Can you work these out from the model? Positions are in its coordinate system, mm. Face numbers are marked on the shaded views. A direction names the side the tool comes from. Round coordinates to 2 decimals unless told otherwise and drop trailing zeros. Order: outer loops, then holes, each group sorted by start corner. A loop starts at its lowest first (then second) coordinate and runs counter-clockwise, first axis right, second up. Notation, with made-up numbers: (4, 74) -> (53, 74) arc R31 ccw to (53, 102) -> close; hole circle Ø10 at (83, 36). An arc over 180 degrees is marked (long way). Use a Markdown table: item, result. Add a question column.
Q1. I need wall thicknesses on line 1 along X through (y, z) = (-21, 76.5); line 2 along Y through (x, z) = (-71, 7.5); line 3 along Y through (x, z) = (-9, 32). Which ranges of each line are inside material? Lowest first, please. Write a range as [from, to].
Q2. If we section it at C-C on y = -6.5: List the corners of the cut face in (x, z) for me, plus the area to 3 significant figures.
Q3. If we section it at B-B on x = -47.5: List the corners of the cut face in (y, z) for me, plus the area to 3 significant figures.
Q4. I'm going to push flat-ended pins straight in: pin 1 Ø5.5 at (x, y) = (0.5, 12) entering from +Z; pin 2 Ø1.5 at (y, z) = (6.5, 69.5) entering from -X; pin 3 Ø5 at (x, z) = (-62.5, 67.5) entering from -Y; pin 4 Ø8 at (x, z) = (-16, 45.5) entering from -Y. Where does each tip first touch, or does it pass through?
Q5. If we section it at A-A on z = 19.5: List the corners of the cut face in (x, y) for me.
Q6. For the marked faces 1 and 2, which set-ups out of +Z, -Z, +X, -X, +Y, -Y let a thin tool reach every point of the face, with its end or its side?
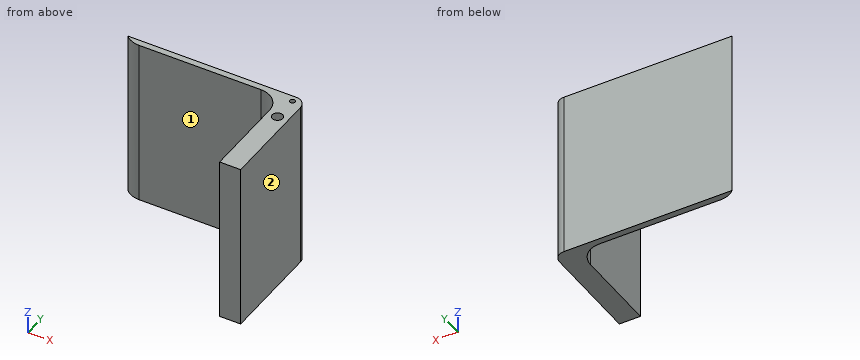
```python
from build123d import *

# Parameters (mm, degrees)
RESSALTO_EXTRUS_O1_DEPTH = 80
ESBO_O3_R                = 2.5
CORTE_EXTRUS_O2_DEPTH    = 10
ESBO_O4_R                = 1.25
CORTE_EXTRUS_O3_DEPTH    = 10
FILETE1_R                = 10
FILETE2_R                = 5
FILETE3_R                = 10


with BuildPart() as part:
    # Esboço1 → Ressalto-extrusão1 (new body)
    with BuildSketch(Plane.XY):
        Polygon((-78.698181647, 27.74137931), (6.301818353, 27.74137931), (6.301818353, 24.74137931), (6.301818353, -25.25862069), (-3.698181647, -25.25862069), (-3.698181647, 24.74137931), (-78.698181647, 24.74137931), align=None)
    extrude(amount=RESSALTO_EXTRUS_O1_DEPTH)

    # Esboço3 → Corte-extrusão2 (cut)
    with BuildSketch(Plane.XY.offset(80)):
        with Locations((1.301818353, 12.74137931)):
            Circle(ESBO_O3_R)
    extrude(amount=-CORTE_EXTRUS_O2_DEPTH, mode=Mode.SUBTRACT)

    # Esboço4 → Corte-extrusão3 (cut)
    with BuildSketch(Plane.XY.offset(80)):
        with Locations((1.301818353, 24.74137931)):
            Circle(ESBO_O4_R)
    extrude(amount=-CORTE_EXTRUS_O3_DEPTH, mode=Mode.SUBTRACT)

    # Filete1
    filete1_edges = [part.edges().sort_by_distance(p)[0] for p in [
        (-3.698181647, 24.74137931, 40),
    ]]
    fillet(filete1_edges, radius=FILETE1_R)

    # Filete2
    filete2_edges = [part.edges().sort_by_distance(p)[0] for p in [
        (6.301818353, 27.74137931, 40),
    ]]
    fillet(filete2_edges, radius=FILETE2_R)

    # Filete3
    # the kernel refuses this fillet: 10 mm, written as the material it takes off along each edge
    with BuildSketch(Plane(origin=(-78.698181647, 24.74137931, -17.853571071), x_dir=(0, 1, 0), z_dir=(0, 0, 1))) as filete3_piece_1:
        with BuildLine():
            CenterArc((10, -7.141428429), FILETE3_R, 134.427004001, 45.572995999)
            Line((0, -7.141428429), (-0.2, -7.141428429))
            Line((-0.2, -7.141428429), (-0.2, 0))
            Line((-0.2, 0), (0, 0.2))
            ThreePointArc((0, 0.2), (1.5, 0.2), (2.86, 0.142828569))
            Line((2.86, 0.142828569), (3, 0))
        make_face()
    extrude(amount=115.707142143, mode=Mode.SUBTRACT)


solid = part.part
```
Answer below:
| question | item | result |
|---|---|---|
| 1 | line 1 | [-3.7, 6.3] |
| 1 | line 2 | [24.74, 27.74] |
| 1 | line 3 | [23.57, 27.74] |
| 2 | outline | (-3.7, 0) -> (6.3, 0) -> (6.3, 80) -> (-3.7, 80) -> close |
| 2 | area | 800 mm² |
| 3 | outline | (24.74, 0) -> (27.74, 0) -> (27.74, 80) -> (24.74, 80) -> close |
| 3 | area | 240 mm² |
| 4 | pin 1 | z = 80 |
| 4 | pin 2 | x = -3.7 |
| 4 | pin 3 | y = 24.74 |
| 4 | pin 4 | y = 24.6 |
| 5 | outline | (-78.7, 27.74) arc R10 ccw to (-71.56, 24.74) -> (-13.7, 24.74) arc R10 cw to (-3.7, 14.74) -> (-3.7, -25.26) -> (6.3, -25.26) -> (6.3, 22.74) arc R5 ccw to (1.3, 27.74) -> close |
| 6 | face 1 | +Z, -Z, -X, -Y |
| 6 | face 2 | +Z, -Z, +X, +Y, -Y |
